Autodesk Inventor part; units mm, degrees
ref_plane "YZ Plane" through (0, 0, 0) normal (1, 0, 0) x (0, 1, 0)
ref_plane "XZ Plane" through (0, 0, 0) normal (0, 1, 0) x (-1, 0, 0)
ref_plane "XY Plane" through (0, 0, 0) normal (0, 0, 1) x (1, 0, 0)
sketch "Sketch1" plane through (0, 0, 0) normal (1, 0, 0) x (0, 1, 0)
  circle A0 centre (0, 0) radius 25.4
  dimension "d0" = 50.8
extrude "Extrusion1" add sketch "Sketch1" along normal blind 34.544
sketch "Sketch2" plane through (34.544, 0, 0) normal (1, 0, 0) x (0, 0, -1)
  circle A0 centre (0, 0) radius 21.082
  dimension "d3" = 42.164
extrude "Extrusion2" add sketch "Sketch2" along normal blind 54.61
sketch "Sketch3" plane through (0, 0, 0) normal (-1, 0, 0) x (0, 0, 1)
  circle A0 centre (0, 8.3566) radius 3.175
  line L0 (0, 0) -> (0, 8.3566) construction
  circle A1 centre (0, 0) radius 25.4
  dimension "d9" = 6.35
  dimension "d10" = 8.3566
extrude "Extrusion3" cut sketch "Sketch3" against normal blind 19.05 contours A0
properties part number "Motor"
Geometry check sheet. Reference: the model listing, model coordinates, mm. A direction names the side the tool comes from. Coordinates: 2 decimals unless noted, no trailing zeros. Order: outer loops, then holes, each group sorted by start corner. A loop starts at its lowest first (then second) coordinate and runs counter-clockwise, first axis right, second up.
Q1. Sectioned sample at D-D on x = 80. Record the cut outline in (y, z).
Reply:
outline: circle Ø42.16 at (0, 0)
Q2. Sectioned sample at B-B on y = -6.5. Record the cut outline in (x, z).
Reply:
outline: (0, -24.55) - (34.54, -24.55) - (34.54, -20.05) - (89.15, -20.05) - (89.15, 20.05) - (34.54, 20.05) - (34.54, 24.55) - (0, 24.55) - close
Q3. Sectioned sample at C-C on x = 6.5. Record the cut outline in (y, z) (3 decimals), and give its area (3 significant figures).
Reply:
outline: circle Ø50.8 at (0, 0); hole circle Ø6.35 at (8.357, 0)
area: 2,000 mm2
Q4. Depth check by flat-ended pin: pin 1 Ø6 at (x, z) = (66, 13) entering from +Y; pin 2 Ø2 at (x, y) = (35, -12.5) entering from -Z; pin 3 Ø1 at (x, z) = (75, -3.5) entering from +Y. Enter the tip coordinate at first touch or a pass-through.
Reply:
pin 1: stops at y = 18.56
pin 2: stops at z = -22.59
pin 3: stops at y = 20.87
Q5. Draft check along Z on faces 3 (the face through (9.392, 5.257, -0.688)), 4 (the face through (34.544, -10, 19)), 5 (the face through (61.47, -6.33, -20.11)). Enter one of: released by +Z, released by -Z, zero draft, split by the parting line, or undercut.
Reply:
face 3: undercut
face 4: zero draft
face 5: split by the parting line
Q6. Thickness scan on probe 1 along X at (y, z) = (-5.5, -21); probe 2 along Z at (x, y) = (23, -10); probe 3 along Z at (x, y) = (77.5, -2). Record the ranges inside material, lowest first.
Reply:
probe 1: x = 0 to 34.54
probe 2: z = -23.35 to 23.35
probe 3: z = -20.99 to 20.99
Q7. Tool access check on faces 1 (the face through (19.05, 8, 0)), 2 (the face through (0, 0, 0)). Record the directions out of +Z, -Z, +X, -X, +Y, -Y that give a thin tool (end or side, any length) a straight path to the whole face; none if there is none.
Reply:
face 1: -X
face 2: +Z, -Z, -X, +Y, -Y
Q8. Sectioned sample at A-A on z = 0. Record the cut outline in (x, y), and give its area (3 significant figures).
Reply:
outline: (0, -25.4) - (34.54, -25.4) - (34.54, -21.08) - (89.15, -21.08) - (89.15, 21.08) - (34.54, 21.08) - (34.54, 25.4) - (0, 25.4) - (0, 11.53) - (19.05, 11.53) - (19.05, 5.18) - (0, 5.18) - close
area: 3,940 mm2
